Geometry check sheet. Reference: the model listing, model coordinates, mm. Face numbers are marked on the shaded views. A direction names the side the tool comes from. Round coordinates to 2 decimals unless told otherwise and drop trailing zeros. Write each loop counter-clockwise with the first axis right and the second up, starting at its lowest first coordinate (ties: lowest second). Pieces come first, ordered by that corner, then holes. Notation, with made-up numbers: M 28,62.25 L 54,62.25 A24 ccw 54,72.25 Z; hole C -3.75,-30 d9. An arc over 180 degrees is marked long. Put each result on its own line as item: value. Start each with the question number.
(1) Section check D-D on z = 2.25. Record the cut outline in (x, y), then the cut area to 3 significant figures.
(2) Section check B-B on x = 4.8. Record the cut outline in (y, z) (3 decimals).
(3) Mould release check, pull along Z, two halves, no side actions. Record for the marked faces 3, 4 and 5: pulls with the +Z half, pulls with the -Z half, needs draft (parallel to the pull), parting line crosses it, or undercut.
(4) Tool access check on the marked faces 1 and 2. Record the directions out of +Z, -Z, +X, -X, +Y, -Y that give a thin tool (end or side, any length) a straight path to the whole face; none if there is none.
(5) Section check A-A on z = 4. Record the cut outline in (x, y) (3 decimals), then the cut area to 3 significant figures.
(6) Material ranges on probe 1 along Y at (x, z) = (7.75, 1.25); probe 2 along Y at (x, z) = (8, 5.25); probe 3 along Z at (x, y) = (5.25, 5.75), recorded low to high.
(7) Section check C-C on y = 5.5. Record the cut outline in (x, z).
(8) Gauge pin test, flat ends, axial feed: pin 1 (1 mm diameter, centred on x = 12, z = 4, fed in from -Y); pin 2 (1.5 mm diameter, centred on x = 12.5, y = 3.5, fed in from -Z); pin 3 (2 mm diameter, centred on x = -4, z = 3.5, fed in from +Y). Record the tip position at first contact, or that the pin passes through.
from build123d import *

# Parameters (mm, degrees)
SKETCH1_W           = 9.6
SKETCH1_H           = 8
BOSS_EXTRUDE1_DEPTH = 4
SKETCH2_R           = 3.5
BOSS_EXTRUDE2_DEPTH = 2
SKETCH3_R           = 2.225
BOSS_EXTRUDE3_DEPTH = 1.9
BOSS_EXTRUDE4_START = -2
SKETCH4_W           = 5.092025843
SKETCH4_H           = 2
BOSS_EXTRUDE4_DEPTH = 0.2


with BuildPart() as part:
    # Sketch1 → Boss-Extrude1 (new body)
    with BuildSketch(Plane(origin=(0, 0, 0), x_dir=(1, 0, 0), z_dir=(0, 1, 0))):
        with Locations((4.8, -4)):
            Rectangle(SKETCH1_W, SKETCH1_H)
        with BuildLine():
            Line((0, 0), (0, -8))
            ThreePointArc((0, -8), (-1.2, -4), (0, 0))
        make_face()
        with BuildLine():
            ThreePointArc((9.6, 0), (10.8, -4), (9.6, -8))
            Line((9.6, -8), (9.6, 0))
        make_face()
    extrude(amount=BOSS_EXTRUDE1_DEPTH)

    # Sketch2 → Boss-Extrude2 (add)
    with BuildSketch(Plane(origin=(0, 4, 0), x_dir=(1, 0, 0), z_dir=(0, 1, 0))):
        with Locations((4.8, -4)):
            Circle(SKETCH2_R)
    extrude(amount=BOSS_EXTRUDE2_DEPTH)

    # Sketch3 → Boss-Extrude3 (add)
    with BuildSketch(Plane(origin=(0, 6, 0), x_dir=(1, 0, 0), z_dir=(0, 1, 0))):
        with Locations((4.8, -4)):
            Circle(SKETCH3_R)
    extrude(amount=BOSS_EXTRUDE3_DEPTH)

    # Sketch4 → Boss-Extrude4 (add)
    with BuildSketch(Plane(origin=(0, 4, 0), x_dir=(1, 0, 0), z_dir=(0, 1, 0)).offset(BOSS_EXTRUDE4_START)):
        with Locations((-3.414000557, -4)):
            Rectangle(SKETCH4_W, SKETCH4_H)
        with Locations((13.014000557, -4)):
            Rectangle(SKETCH4_W, SKETCH4_H)
    extrude(amount=BOSS_EXTRUDE4_DEPTH)


solid = part.part
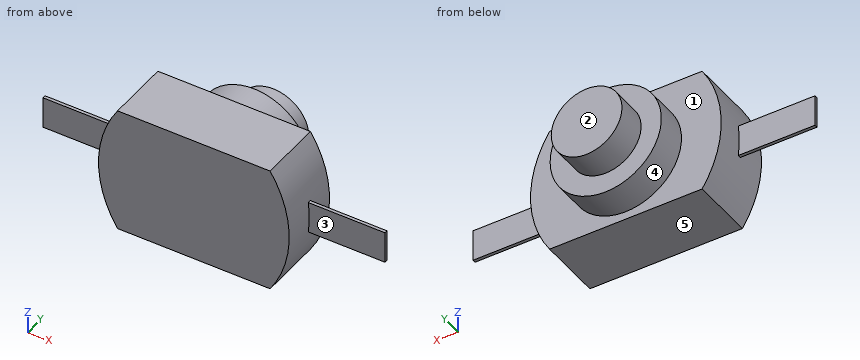
Answers follow:
1. outline: M -0.99,0 L 10.59,0 L 10.59,4 L 7.83,4 L 7.83,6 L 6.17,6 L 6.17,7.9 L 3.43,7.9 L 3.43,6 L 1.77,6 L 1.77,4 L -0.99,4 Z
1. area: 63.6 mm^2
2. outline: M 0,0 L 4,0 L 4,0.5 L 6,0.5 L 6,1.775 L 7.9,1.775 L 7.9,6.225 L 6,6.225 L 6,7.5 L 4,7.5 L 4,8 L 0,8 Z
3. face 3: needs draft
3. face 4: parting line crosses it
3. face 5: pulls with the -Z half
4. face 1: +Y
4. face 2: +Z, -Z, +X, -X, +Y
5. outline: M -5.96,2 L -1.2,2 L -1.2,0 L 10.8,0 L 10.8,2 L 15.56,2 L 15.56,2.2 L 10.8,2.2 L 10.8,4 L 8.3,4 L 8.3,6 L 7.025,6 L 7.025,7.9 L 2.575,7.9 L 2.575,6 L 1.3,6 L 1.3,4 L -1.2,4 L -1.2,2.2 L -5.96,2.2 Z
5. area: 72.4 mm^2
6. probe 1: y = 0 to 4
6. probe 2: y = 0 to 6
6. probe 3: z = 0.53 to 7.47
7. outline: C 4.8,4 d7
8. pin 1: stops at y = 2
8. pin 2: passes through
8. pin 3: stops at y = 2.2
